Geometry check sheet. Reference: the model listing, model coordinates, mm. A direction names the side the tool comes from. Coordinates: 2 decimals unless noted, no trailing zeros. Order: outer loops, then holes, each group sorted by start corner. A loop starts at its lowest first (then second) coordinate and runs counter-clockwise, first axis right, second up. Notation, with made-up numbers: (-14, -35.5) - (34, -35.5) arc R26 cw to (34, -7.5) - close; hole circle Ø10 at (30, 61). An arc over 180 degrees is marked (long way). Return JSON: item names as keys, results as strings. Group by question number.
Item 1: Section check B-B on z = 13.5. Enter the section's corners in (x, y), then the cut area to 3 significant figures.
Item 2: Section check C-C on x = -0.25. Enter the section's corners in (y, z).
Item 3: Tool access check on faces 1 (the flat face through (0, 230, 25)), 2 (the flat face through (-4.35, 108.46, 2.465)), 3 (the flat face through (0, 225, 17)), 4 (the flat face through (4.31, 108.46, 2.535)), 5 (the cylindrical face through (-0.04, 230.49, -0.72)). Record the directions out of +Z, -Z, +X, -X, +Y, -Y that give a thin tool (end or side, any length) a straight path to the whole face; none if there is none.
Item 4: Scan lines: probe 1 along Z at (x, y) = (-2, 131.5); probe 2 along Y at (x, z) = (-0.25, 19.5); probe 3 along X at (y, z) = (84, -1). Record each from-to range of solid material in increasing order.
Item 5: Gauge pin test, flat ends, axial feed: pin 1 (1.7 mm diameter, centred on x = 0, z = 18.5, fed in from -Y); pin 2 (6.5 mm diameter, centred on x = 1, y = 123.5, fed in from +Z); pin 3 (2 mm diameter, centred on x = -1, z = 1, fed in from +Y). Record the tip position at first contact, or that the pin passes through.
Item 6: Section check A-A on y = 22.5. Enter the section's corners in (x, z).
from build123d import *

# Parameters (mm, degrees)
BOSS_EXTRUDE1_DEPTH = 220
REVOLVE1_ANGLE      = 90
BOSS_EXTRUDE2_DEPTH = 15


with BuildPart() as part:
    # Sketch1 → Boss-Extrude1 (new body)
    with BuildSketch(Plane(origin=(0, 0, 0), x_dir=(1, 0, 0), z_dir=(0, 1, 0))):
        Polygon((5.773502692, 0), (2.886751346, 5), (-2.886751346, 5), (-5.773502692, 0), (-2.886751346, -5), (2.886751346, -5), align=None)
    extrude(amount=BOSS_EXTRUDE1_DEPTH)

    # Sketch2 → Revolve1 (revolve)
    with BuildSketch(Plane(origin=(0, 220, 0), x_dir=(1, 0, 0), z_dir=(0, 1, 0))):
        Polygon((-2.886751346, -5), (2.886751346, -5), (5.773502692, 0), (2.886751346, 5), (-2.886751346, 5), (-5.773502692, 0), align=None)
    revolve(axis=Axis((-6.610252502, 220, 10), (1, 0, 0)), revolution_arc=REVOLVE1_ANGLE)

    # Sketch3 → Boss-Extrude2 (add)
    with BuildSketch(Plane.XY.offset(10)):
        Polygon((-5.773502692, 230), (-2.886751346, 225), (2.886751346, 225), (5.773502692, 230), (2.886751346, 235), (-2.886751346, 235), align=None)
    extrude(amount=BOSS_EXTRUDE2_DEPTH)


solid = part.part
Computed:
{
 "1": {"outline": "(-5.77, 230) - (-2.89, 225) - (2.89, 225) - (5.77, 230) - (2.89, 235) - (-2.89, 235) - close", "area": "86.6 mm²"},
 "2": {"outline": "(0, -5) - (220, -5) arc R15 ccw to (235, 10) - (235, 25) - (225, 25) - (225, 10) arc R5 cw to (220, 5) - (0, 5) - close"},
 "3": {"face 1": "+Z, +X, -X, +Y, -Y", "face 2": "+Z, -X, -Y", "face 3": "+Z, +X, -X, -Y", "face 4": "+Z, +X, -Y", "face 5": "-Z, +X, -X, +Y"},
 "4": {"probe 1": "z = -5 to 5", "probe 2": "y = 225 to 235", "probe 3": "x = -5.2 to 5.2"},
 "5": {"pin 1": "stops at y = 225", "pin 2": "stops at z = 5", "pin 3": "stops at y = 232.69"},
 "6": {"outline": "(-5.77, 0) - (-2.89, -5) - (2.89, -5) - (5.77, 0) - (2.89, 5) - (-2.89, 5) - close"}
}
